```python
from build123d import *

# Parameters (mm, degrees)
BOSS_EXTRUDE1_DEPTH = 1.6
SKETCH8_3_R         = 2.5
CUT_EXTRUDE1_DEPTH  = 178.756608161
SKETCH25_R          = 2.5
CUT_EXTRUDE2_DEPTH  = 178.756608161
CUT_EXTRUDE3_DEPTH  = 175.275284078


with BuildPart() as part:
    # Sketch8 → Boss-Extrude1 (new body)
    with BuildSketch(Plane.XY):
        with BuildLine():
            ThreePointArc((103.534701401, 106.398987898), (103.693161759, 110.090138371), (104.446158593, 113.707139515))
            ThreePointArc((104.446158593, 113.707139515), (97.535722451, 128.659745128), (81.803110207, 123.779227301))
            ThreePointArc((81.803110207, 123.779227301), (68.396685685, 109.506582784), (50.436082024, 101.705472858))
            ThreePointArc((50.436082024, 101.705472858), (40.732585656, 91.888172428), (45.984244445, 79.122699094))
            ThreePointArc((45.984244445, 79.122699094), (60.856228216, 70.93053968), (76.976923111, 65.600382715))
            ThreePointArc((76.976923111, 65.600382715), (77.137220348, 65.563882378), (77.2977589, 65.528458486))
            ThreePointArc((77.2977589, 65.528458486), (77.354298773, 65.515492739), (77.410522602, 65.501218676))
            ThreePointArc((77.410522602, 65.501218676), (94.023303804, 63.303193357), (110.759742778, 64.144278965))
            ThreePointArc((110.759742778, 64.144278965), (121.287127646, 74.212620667), (115.130462452, 87.414620912))
            ThreePointArc((115.130462452, 87.414620912), (112.067901623, 89.481121015), (109.379631064, 92.015465685))
            ThreePointArc((109.379631064, 92.015465685), (109.377986421, 92.015505684), (109.376341775, 92.015545509))
            ThreePointArc((109.376341775, 92.015545509), (109.37615287, 92.017539878), (109.375963817, 92.019534234))
            ThreePointArc((109.375963817, 92.019534234), (105.194093866, 98.693961054), (103.534911629, 106.393514545))
            ThreePointArc((103.534911629, 106.393514545), (103.533655951, 106.395075463), (103.532400156, 106.396636288))
            ThreePointArc((103.532400156, 106.396636288), (103.533550841, 106.397812032), (103.534701401, 106.398987898))
        make_face()
    extrude(amount=BOSS_EXTRUDE1_DEPTH)

    # Sketch8<3> → Cut-Extrude1 (cut, through all)
    with BuildSketch(Plane.XY):
        with Locations((70.435309654, 103.157249982)):
            Circle(SKETCH8_3_R)
    extrude(amount=CUT_EXTRUDE1_DEPTH, mode=Mode.SUBTRACT)

    # Sketch25 → Cut-Extrude2 (cut, through all)
    with BuildSketch(Plane.XY):
        with Locations((84.959968883, 101.629007764)):
            Circle(SKETCH25_R)
        with Locations((62.365539379, 86.956013681)):
            Circle(SKETCH25_R)
        with Locations((80.999251173, 82.99529597)):
            Circle(SKETCH25_R)
        with Locations((99.632962967, 79.03457826)):
            Circle(SKETCH25_R)
    extrude(amount=CUT_EXTRUDE2_DEPTH, mode=Mode.SUBTRACT)

    # Sketch23 → Cut-Extrude3 (cut, through all)
    with BuildSketch(Plane(origin=(-19.097367964, 26.776820286, 0), x_dir=(0.9781476007338056, -0.2079116908177598, 0), z_dir=(0, 0, 1))):
        Polygon((103.223291241, 65.776224437), (91.223291241, 65.776224437), (91.223291241, 59.276224437), (99.703476733, 59.276224437), (103.223291241, 60.67197249), align=None)
    extrude(amount=CUT_EXTRUDE3_DEPTH, mode=Mode.SUBTRACT)


solid = part.part
```
For this review, take the finished solid that the model builds, in its own axes (mm). A direction names the side the tool comes from. Coordinates: 2 decimals unless noted, no trailing zeros. Loops run counter-clockwise (first coordinate to the right, second up) from the corner with the lowest first, then second, coordinate; pieces in that order, holes last. Notation, with made-up numbers: (-20.5, -32.5) - (32.5, -32.5) arc R17 ccw to (32.5, -22.5) - close; hole circle Ø11 at (42.25, 56.25). An arc over 180 degrees is marked (long way). Use one line per item in the form item = value. Start each with the question number.
1) Take a section at C-C (y = 120). State the section outline as (x, z) points.
2) Take a section at D-D (x = 64). State the section outline as (y, z) points.
3) Take a section at B-B (x = 93). State the section outline as (y, z) points.
4) Take a section at A-A (z = 0.25). State how many separate pieces and enclosed holes the cut face has, plus the area to 3 significant figures.
5) Draft analysis for pull direction X (two halves, no side actions). For faces 4 (the face through (93.789, 63.313, 0.789)), 5 (the face through (92.59, 64.34, 0.79)), 6 (the face through (68.622, 109.666, 0.789)), state which applies: released by +X, released by -X, zero draft, split by the parting line, or undercut.
6) For faces 1 (the face through (83.14, 69.01, 0.79)), 2 (the face through (105.236, 98.591, 0.789)), 3 (the face through (80, 90, 0)), list the 3-axis set-ups (+Z, -Z, +X, -X, +Y, -Y) from which the entire face can be reached by the end or side of a thin tool; tool diameter is ignored.
7) To check wall thickness, follow probe 1 along Y at (x, z) = (86.5, 0.1); probe 2 along X at (y, z) = (87, 1.4); probe 3 along X at (y, z) = (84, 1.35). State the ranges of each line that lie inside material, in increasing order. Write a range as from..to.
8) For pin 1 (4.5 mm diameter, centred on x = 70.44, y = 103.16, fed in from +Z), flat-tipped, find the tip position at first contact; note if it passes through.
From the geometry:
q1.outline = (79.23, 0) - (104.65, 0) - (104.65, 1.6) - (79.23, 1.6) - close
q2.outline = (69.63, 0) - (85.06, 0) - (85.06, 1.6) - (69.63, 1.6) - close; (88.85, 0) - (106.75, 0) - (106.75, 1.6) - (88.85, 1.6) - close
q3.outline = (63.35, 0) - (64.41, 0) - (64.41, 1.6) - (63.35, 1.6) - close; (70.2, 0) - (129.73, 0) - (129.73, 1.6) - (70.2, 1.6) - close
q4.separate_pieces = 1
q4.enclosed_holes = 6
q4.area = 3,110 mm2
q5.face_4 = split by the parting line
q5.face_5 = undercut
q5.face_6 = released by -X
q6.face_1 = +Z, -Z
q6.face_2 = +Z, -Z, +X
q6.face_3 = -Z, +X, -X, +Y, -Y
q7.probe_1 = 63.92..64.93, 71.58..99.66, 103.6..128.23
q7.probe_2 = 40.74..59.87, 64.87..115.82
q7.probe_3 = 41.76..78.71, 83.29..119.02
q8.pin_1 = through
